Could you check a few things on this model? Use its own coordinates, in mm. Face numbers are marked on the shaded views. A direction names the side the tool comes from. Round coordinates to 2 decimals unless told otherwise and drop trailing zeros. Write each loop counter-clockwise with the first axis right and the second up, starting at its lowest first coordinate (ties: lowest second). Pieces come first, ordered by that corner, then holes.
```python
from build123d import *

# Parameters (mm, degrees)
F1_DEPTH = 15.24
F2_DEPTH = 10.16
F0_W     = 4.953
F0_H     = 11.6882068259
F0_W_2   = 7.8621185967
F3_DEPTH = 10.16
F4_DEPTH = 3.81


# Not quite as in the source:
# - a feature names something its author has since deleted; it is built from what else it names


with BuildPart() as f1:
    # F0 (on Top) → F1 (new body)
    with BuildSketch(Plane.XY):
        Polygon((56.8358146836, 36.3690045497), (31.4358146836, 36.3690045497), (4.7581588602, 91.852396227), (-21.9194969632, 36.3690045497), (-23.4601999485, 36.3690045497), (-47.3194969632, 36.3690045497), (-63.1618590029, 3.4205332163), (-65.7835588108, -2.0319997298), (-60.7738408696, -2.0319997298), (-60.7738408696, -52.8319997298), (70.29015859, -52.8319997298), (70.29015859, -2.0319997298), (75.2998765312, -2.0319997298), (72.6781767233, 3.4205332163), align=None)
        Polygon((68.2581588602, -50.8), (-58.7418411398, -50.8), (-58.7418411398, 0), (-62.5518411398, 0), (-61.8190678495, 1.524), (-46.0418411398, 34.3370048199), (-22.332856425, 34.3370048199), (-20.6418411398, 34.3370048199), (-18.376729311, 39.0479167388), (-8.5820728345, 59.4185506966), (-6.3910428531, 63.9753894023), (4.7581588602, 87.1631660812), (15.9073605735, 63.9753894023), (18.0983905549, 59.4185506966), (27.8930470314, 39.0479167388), (30.1581588602, 34.3370048199), (31.8491741455, 34.3370048199), (55.5581588602, 34.3370048199), (71.3353855699, 1.524), (72.0681588602, 0), (68.2581588602, 0), align=None, mode=Mode.SUBTRACT)
    extrude(amount=F1_DEPTH)

    # F0 (on Top) → F2 (join)
    with BuildSketch(Plane.XY):
        Polygon((-62.5518411398, 0), (-58.7418411398, 0), (-33.3418411398, 0), (-36.0511744731, 2.2891336547), (-32.5333754715, 9.6053469359), (-30.7009610057, 13.4163478047), (-20.6418411398, 34.3370048199), (-22.332856425, 34.3370048199), (-38.1100831348, 1.524), (-58.7418411398, 1.524), (-61.8190678495, 1.524), align=None)
        Polygon((42.8581588602, 0), (68.2581588602, 0), (72.0681588602, 0), (71.3353855699, 1.524), (68.2581588602, 1.524), (47.6264008552, 1.524), (31.8491741455, 34.3370048199), (30.1581588602, 34.3370048199), (40.2172787262, 13.4163478047), (42.0496931919, 9.6053469359), (45.5674921935, 2.2891336547), align=None)
    extrude(amount=F2_DEPTH)



with BuildPart() as f3:
    # F0 (on Top) → F3 (new body)
    with BuildSketch(Plane.XY):
        Polygon((-6.1638411398, 34.3370048199), (-6.1638411398, 13.4163478047), (-5.1478411398, 13.4163478047), (-5.1478411398, 25.1078879876), (-0.1948411398, 25.1078879876), (-0.1948411398, 13.4163478047), (0.8297724999, 13.4163478047), (0.8297724999, 25.1078879876), (8.6918910965, 25.1078879876), (8.6918910965, 13.4163478047), (9.7111588602, 13.4163478047), (9.7111588602, 25.1078879876), (14.6641588602, 25.1078879876), (14.6641588602, 13.4163478047), (15.6801588602, 13.4163478047), (15.6801588602, 34.3370048199), (15.6801588602, 39.0479167388), (5.8855023837, 59.4185506966), (4.7581588602, 59.4185506966), (3.6308153367, 59.4185506966), (-6.1638411398, 39.0479167388), align=None)
        with Locations((-2.6713411398, 31.9604512176)):
            Rectangle(F0_W, F0_H, mode=Mode.SUBTRACT)
        Polygon((-5.1478411398, 38.8163478047), (-0.1948411398, 49.1174492506), (-0.1948411398, 38.8163478047), align=None, mode=Mode.SUBTRACT)
        with Locations((4.7608317982, 31.9604512176)):
            Rectangle(F0_W_2, F0_H, mode=Mode.SUBTRACT)
        with Locations((12.1876588602, 31.9604512176)):
            Rectangle(F0_W, F0_H, mode=Mode.SUBTRACT)
        Polygon((9.7111588602, 49.1174492506), (14.6641588602, 38.8163478047), (9.7111588602, 38.8163478047), align=None, mode=Mode.SUBTRACT)
        Polygon((0.8297724999, 51.2484100915), (4.7581588602, 59.4185506966), (8.6918910965, 51.2372918984), (8.6918910965, 38.8163478047), (0.8297724999, 38.8163478047), align=None, mode=Mode.SUBTRACT)
        Polygon((4.7581588602, 61.7631660812), (3.6308153367, 59.4185506966), (4.7581588602, 59.4185506966), (5.8855023837, 59.4185506966), align=None)
        Polygon((-5.1478411398, 13.4163478047), (-6.1638411398, 13.4163478047), (-6.1638411398, 12.4003478047), (15.6801588602, 12.4003478047), (15.6801588602, 13.4163478047), (14.6641588602, 13.4163478047), (9.7111588602, 13.4163478047), (8.6918910965, 13.4163478047), (0.8297724999, 13.4163478047), (-0.1948411398, 13.4163478047), align=None)
    extrude(amount=F3_DEPTH)


with BuildPart() as f1_1:
    add(f1.part)

    add(f3.part)  # F4 merges F3
    # F0 (on Top) → F4 (join)
    with BuildSketch(Plane.XY):
        Polygon((-30.7009610057, 13.4163478047), (-32.5333754715, 9.6053469359), (42.0496931919, 9.6053469359), (40.2172787262, 13.4163478047), (15.6801588602, 13.4163478047), (15.6801588602, 12.4003478047), (-6.1638411398, 12.4003478047), (-6.1638411398, 13.4163478047), align=None)
        Polygon((-18.376729311, 39.0479167388), (-20.6418411398, 34.3370048199), (-6.1638411398, 34.3370048199), (-6.1638411398, 39.0479167388), align=None)
        Polygon((15.6801588602, 34.3370048199), (30.1581588602, 34.3370048199), (27.8930470314, 39.0479167388), (15.6801588602, 39.0479167388), align=None)
        Polygon((-6.3910428531, 63.9753894023), (-8.5820728345, 59.4185506966), (3.6308153367, 59.4185506966), (4.7581588602, 61.7631660812), (5.8855023837, 59.4185506966), (18.0983905549, 59.4185506966), (15.9073605735, 63.9753894023), align=None)
    extrude(amount=F4_DEPTH)


solid = f1_1.part
```
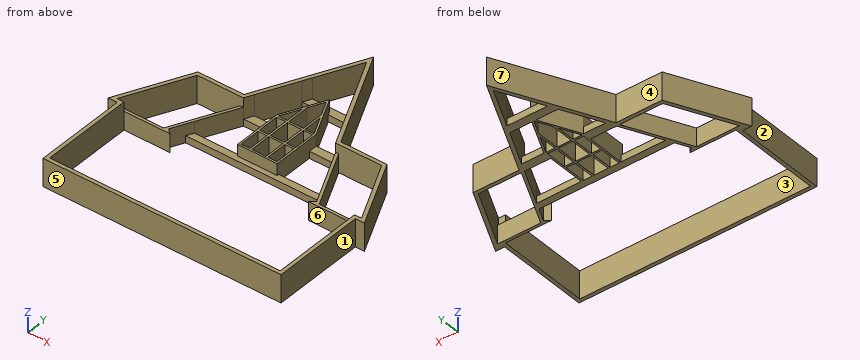
Q1. We'd pull the mould along Y, two halves only. Please class the marked faces 5, 6 and 7: pulls with the +Y half, pulls with the -Y half, needs draft (parallel to the pull), parting line crosses it, or undercut.
Q2. Imagine slicing it at D-D, the plane y = 53. Write out the boundary of the cut face in (x, z), then the cut area to 3 significant figures.
Q3. Imagine slicing it at C-C, the plane z = 13.5. Write out the boundary of the cut face in (x, y), then the cut area to 3 significant figures.
Q4. If I drill on L1, parallel to Y at x = 55.5, z = 2.25; L2, parallel to Y at x = -39.5, z = 12.25; L3, parallel to Y at x = 66, z = 6, over which ranges is the centre line in solid material (lowest first)?
Q5. I'm going to push flat-ended pins straight in: pin 1 Ø5 at (y, z) = (29.5, 3.5) entering from -X; pin 2 Ø4 at (y, z) = (-10, 2) entering from -X; pin 3 Ø3 at (y, z) = (17, 6) entering from -X. Where does each tip first touch, or does it pass through?
Q6. On a 3-axis mill with a long thin cutter (end or side, diameter ignored), from which of +Z, -Z, +X, -X, +Y, -Y can I reach the whole of each face in a straight line? I mean the marked faces 1, 2, 3 and 4. Say none if no direction works.
Q7. Imagine slicing it at A-A, the plane y = -28.5. Write out the boundary of the cut face in (x, z).
Q8. Imagine slicing it at B-B, the plane x = -42. Write out the boundary of the cut face in (y, z), then the cut area to 3 significant figures.
Results found:
1. face 5: pulls with the -Y half
1. face 6: undercut
1. face 7: pulls with the +Y half
2. outline: (-13.92, 0) - (-11.67, 0) - (-11.67, 15.24) - (-13.92, 15.24) - close; (0.54, 0) - (1.67, 0) - (1.67, 10.16) - (0.54, 10.16) - close; (7.84, 0) - (8.97, 0) - (8.97, 10.16) - (7.84, 10.16) - close; (21.18, 0) - (23.44, 0) - (23.44, 15.24) - (21.18, 15.24) - close
2. area: 91.6 mm2
3. outline: (-65.78, -2.03) - (-60.77, -2.03) - (-60.77, -52.83) - (70.29, -52.83) - (70.29, -2.03) - (75.3, -2.03) - (56.84, 36.37) - (31.44, 36.37) - (4.76, 91.85) - (-21.92, 36.37) - (-47.32, 36.37) - close; hole (-62.55, 0) - (-58.74, 0) - (-58.74, -50.8) - (68.26, -50.8) - (68.26, 0) - (72.07, 0) - (55.56, 34.34) - (30.16, 34.34) - (4.76, 87.16) - (-20.64, 34.34) - (-46.04, 34.34) - close
3. area: 998 mm2
4. L1: y = -52.83 to -50.8, 0 to 1.52, 34.34 to 36.37
4. L2: y = -52.83 to -50.8, 34.34 to 36.37
4. L3: y = -52.83 to -50.8, 0 to 1.52, 12.62 to 17.31
5. pin 1: stops at x = -51.82
5. pin 2: stops at x = -60.77
5. pin 3: stops at x = -57.35
6. face 1: +Z, -Z, +X, -Y
6. face 2: +Z, -Z, -X, -Y
6. face 3: +Z, -Z
6. face 4: +Z, -Z, -X, +Y
7. outline: (-60.77, 0) - (-58.74, 0) - (-58.74, 15.24) - (-60.77, 15.24) - close; (68.26, 0) - (70.29, 0) - (70.29, 15.24) - (68.26, 15.24) - close
8. outline: (-52.83, 0) - (-50.8, 0) - (-50.8, 15.24) - (-52.83, 15.24) - close; (0, 0) - (1.52, 0) - (1.52, 10.16) - (0, 10.16) - close; (34.34, 0) - (36.37, 0) - (36.37, 15.24) - (34.34, 15.24) - close
8. area: 77.4 mm2
